```python
from build123d import *

# Parameters (mm, degrees)
F0_R     = 38.1
F0_R_2   = 32.0675
F1_DEPTH = 63.5
F2_DEPTH = 6.35
F3_R     = 4.7625
F4_DEPTH = 25.4
F5_R     = 63.5
F6_DEPTH = 25.4
F7_R     = 12.7
F7_R_2   = 25.4
F8_DEPTH = 12.7


with BuildPart() as f1:
    # F0 (on Top) → F1 (new body)
    with BuildSketch(Plane.XY):
        Circle(F0_R)
        Circle(F0_R_2, mode=Mode.SUBTRACT)
        Circle(F0_R_2)
    extrude(amount=F1_DEPTH)

    # F0 (on Top) → F2 (cut)
    with BuildSketch(Plane.XY):
        Circle(F0_R_2)
    extrude(amount=F2_DEPTH, mode=Mode.SUBTRACT)

    # F3 (on Top) → F4 (cut)
    with BuildSketch(Plane.XY):
        Circle(F3_R)
    extrude(amount=F4_DEPTH, mode=Mode.SUBTRACT)

    # F5 (on face) → F6 (join)
    with BuildSketch(Plane.XY.offset(63.5)):
        Circle(F5_R)
    extrude(amount=F6_DEPTH)

    # F7 (on face) → F8 (cut)
    with BuildSketch(Plane.XY.offset(88.9)):
        with Locations((0, 48.26)):
            Circle(F7_R)
        with Locations((-41.794386, -24.13)):
            Circle(F7_R)
        with Locations((41.794386, -24.13)):
            Circle(F7_R)
        Circle(F7_R_2)
    extrude(amount=-F8_DEPTH, mode=Mode.SUBTRACT)


solid = f1.part
```
Build history of the part. All positions in model axes, mm. A direction names the side the tool comes from. Coordinates: 2 decimals unless noted, no trailing zeros. Write each loop counter-clockwise with the first axis right and the second up, starting at its lowest first coordinate (ties: lowest second). Pieces come first, ordered by that corner, then holes.
1. 3-axis set-ups, long thin cutter, end or side, ignore diameter. For faces 5 (the flat face through (0, 0, 25.4)), 6 (the flat face through (-1, -27, 88.9)), 7 (the cylindrical face through (6.827, 58.969, 82.639)): which of +Z, -Z, +X, -X, +Y, -Y reach the whole face in a straight line?
Answer block:
face 5: -Z
face 6: +Z, +X, -X, +Y, -Y
face 7: +Z
2. Band-saw the part on C-C, the plane x = 0. Give the cut face in (y, z), and give its area (3 significant figures).
Answer block:
outline: (-63.5, 63.5) - (-38.1, 63.5) - (-38.1, 0) - (-32.07, 0) - (-32.07, 6.35) - (-4.76, 6.35) - (-4.76, 25.4) - (4.76, 25.4) - (4.76, 6.35) - (32.07, 6.35) - (32.07, 0) - (38.1, 0) - (38.1, 63.5) - (63.5, 63.5) - (63.5, 88.9) - (60.96, 88.9) - (60.96, 76.2) - (35.56, 76.2) - (35.56, 88.9) - (25.4, 88.9) - (25.4, 76.2) - (-25.4, 76.2) - (-25.4, 88.9) - (-63.5, 88.9) - close
area: 6,510 mm2
3. Band-saw the part on B-B, the plane z = 79. Give the cut face in (x, y).
Answer block:
outline: circle Ø127 at (0, 0); hole circle Ø25.4 at (-41.79, -24.13); hole circle Ø50.8 at (0, 0); hole circle Ø25.4 at (0, 48.26); hole circle Ø25.4 at (41.79, -24.13)
4. Band-saw the part on D-D, the plane x = 22. Give the cut face in (y, z), and give its area (3 significant figures).
Answer block:
outline: (-59.57, 63.5) - (-31.11, 63.5) - (-31.11, 0) - (-23.33, 0) - (-23.33, 6.35) - (23.33, 6.35) - (23.33, 0) - (31.11, 0) - (31.11, 63.5) - (59.57, 63.5) - (59.57, 88.9) - (12.69, 88.9) - (12.69, 76.2) - (-12.69, 76.2) - (-12.69, 88.9) - (-59.57, 88.9) - close
area: 6,360 mm2
5. Band-saw the part on A-A, the plane y = 0. Give the cut face in (x, z).
Answer block:
outline: (-63.5, 63.5) - (-38.1, 63.5) - (-38.1, 0) - (-32.07, 0) - (-32.07, 6.35) - (-4.76, 6.35) - (-4.76, 25.4) - (4.76, 25.4) - (4.76, 6.35) - (32.07, 6.35) - (32.07, 0) - (38.1, 0) - (38.1, 63.5) - (63.5, 63.5) - (63.5, 88.9) - (25.4, 88.9) - (25.4, 76.2) - (-25.4, 76.2) - (-25.4, 88.9) - (-63.5, 88.9) - close
6. Drop flat-ended pins along their axis: pin 1 (2 mm diameter, centred on x = 3, z = 40.5, fed in from -Y); pin 2 (20.5 mm diameter, centred on x = 41.79, y = -24.13, fed in from +Z); pin 3 (1 mm diameter, centred on y = 22, z = 19.5, fed in from +X). Give the stop position or say it passes through.
Answer block:
pin 1: stops at y = -38.05
pin 2: stops at z = 76.2
pin 3: stops at x = 31.45
7. Pull direction X, two halves, no side cores. Call faces 1 (the flat face through (-17, -28, 0)), 2 (the cylindrical face through (-13.77, -61.99, 76.02)), 3 (the flat face through (-42, -24, 76.2)), 4 (the cylindrical face through (-5.506, -24.796, 82.639)): released by +X, released by -X, zero draft, split by the parting line, or undercut.
Answer block:
face 1: zero draft
face 2: split by the parting line
face 3: undercut
face 4: undercut
8. Drill centre lines: probe 1 along Y at (x, z) = (0, 83.75); probe 2 along Z at (x, y) = (-19, 10); probe 3 along X at (y, z) = (3, 13). Where is each one in solid material? Low to high.
Answer block:
probe 1: y = -63.5 to -25.4, 25.4 to 35.56, 60.96 to 63.5
probe 2: z = 6.35 to 76.2
probe 3: x = -37.98 to -3.7, 3.7 to 37.98
